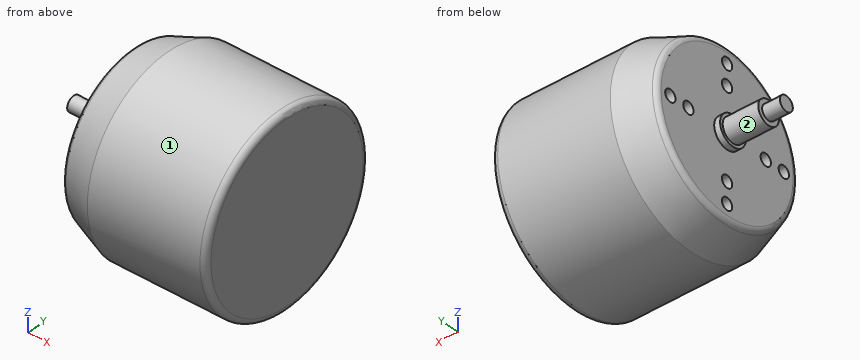
Autodesk Inventor part; units mm, degrees
ref_plane "YZ Plane" through (0, 0, 0) normal (1, 0, 0) x (0, 1, 0)
ref_plane "XZ Plane" through (0, 0, 0) normal (0, 1, 0) x (-1, 0, 0)
ref_plane "XY Plane" through (0, 0, 0) normal (0, 0, 1) x (1, 0, 0)
sketch "Sketch1" plane through (0, 0, 0) normal (0, 0, 1) x (1, 0, 0)
  line L0 (0, 0) -> (0, 27)
  line L1 (0, 0) -> (52, 0)
  line L2 (52, 0) -> (52, 31.5)
  line L3 (52, 31.5) -> (12, 31.5)
  line L4 (12, 31.5) -> (0, 27)
  dimension "d1" = 27
  dimension "d2" = 52
  dimension "d3" = 31.5
  dimension "d4" = 40
revolve "Revolution1" add sketch "Sketch1" angle 360 about axis through (0, 0, 0) along (1, 0, 0)
sketch "Sketch2" plane through (0, 0, 0) normal (-1, 0, 0) x (0, 0, 1)
  circle A0 centre (0, 0) radius 5
  dimension "d6" = 10
extrude "Extrusion1" add sketch "Sketch2" along normal blind 2
sketch "Sketch3" plane through (-2, 0, 0) normal (-1, 0, 0) x (0, 0, 1)
  circle A0 centre (0, 0) radius 4
  dimension "d9" = 8
extrude "Extrusion2" add sketch "Sketch3" along normal blind 12
sketch "Sketch4" plane through (-14, 0, 0) normal (-1, 0, 0) x (0, 0, 1)
  circle A0 centre (0, 0) radius 4
  circle A1 centre (0, 0) radius 2.5
  dimension "d12" = 5
extrude "Extrusion3" add sketch "Sketch4" along normal blind 6 contours A1
thread "Thread1"
thread "Thread2"
fillet "Fillet1" radius 2 2 edges at (0, -27, 0) (52, -31.5, 0)
sketch "Sketch5" plane through (0, 0, 0) normal (-1, 0, 0) x (0, 0, 1)
  circle A0 centre (0, 15) radius 2
  circle A1 centre (0, 22) radius 2
  circle A2 centre (-15, 0) radius 2
  circle A3 centre (-22, 0) radius 2
  circle A4 centre (0, -15) radius 2
  circle A5 centre (0, -22) radius 2
  circle A6 centre (15, 0) radius 2
  circle A7 centre (22, 0) radius 2
  point P0 (0, 0)
  dimension "d20" = 4
  dimension "d21" = 4
  dimension "d24" = 360
extrude "Extrusion4" cut sketch "Sketch5" against normal blind 8
properties part number "moteur"
Design review of the part built by this model. Coordinates are the model's own, in mm. Face numbers are marked on the shaded views. A direction names the side the tool comes from. Round coordinates to 2 decimals unless told otherwise and drop trailing zeros. Write each loop counter-clockwise with the first axis right and the second up, starting at its lowest first coordinate (ties: lowest second). Pieces come first, ordered by that corner, then holes. Notation, with made-up numbers: (46, -1) -> (84, -1) arc R23 cw to (84, 35) -> close; hole circle Ø10 at (20, 20). An arc over 180 degrees is marked (long way). Write item = value, one per line. Start each with the question number.
1) Take a section at B-B, the plane x = 39.5. State the section outline as (y, z) points, plus the area to 3 significant figures.
2) Take a section at A-A, the plane x = 6.5. Count the separate pieces of the cut face and the enclosed holes in it, plus the area to 3 significant figures.
3) Clearance check with flat-ended pins moving along their axes: pin 1 (2.5 mm diameter, centred on y = 22, z = 0, fed in from -X); pin 2 (2 mm diameter, centred on x = 10, y = -3.5, fed in from +Z); pin 3 (4.5 mm diameter, centred on y = 15, z = 0, fed in from -X). State where each tip first meets the part, or that it passes through.
4) Wall thickness on probe 1 along Y at (x, z) = (5.75, 0); probe 2 along X at (y, z) = (-16.5, 12.5); probe 3 along Y at (x, z) = (2, 0): over which ranges is each line inside the solid? List them lowest first. Write a range as from..to.
5) Tool access review of the marked faces 1 and 2: name each direction out of +Z, -Z, +X, -X, +Y, -Y from which nothing blocks a thin tool from reaching the whole face with its end or side.
Results list:
q1.outline = circle Ø63 at (0, 0)
q1.area = 3,120 mm²
q2.separate_pieces = 1
q2.enclosed_holes = 8
q2.area = 2,620 mm²
q3.pin_1 = 8
q3.pin_2 = 30.94
q3.pin_3 = 0
q4.probe_1 = -29.16..-24, -20..-17, -13..13, 17..20, 24..29.16
q4.probe_2 = 0..52
q4.probe_3 = -27.75..-24, -20..-17, -13..13, 17..20, 24..27.75
q5.face_1 = +X, -X
q5.face_2 = -X
